Verification items for the finished model (mm, model axes). Face numbers are marked on the shaded views. A direction names the side the tool comes from. Coordinates: 2 decimals unless noted, no trailing zeros. Loops run counter-clockwise (first coordinate to the right, second up) from the corner with the lowest first, then second, coordinate; pieces in that order, holes last. Notation, with made-up numbers: (88.25, 39) - (107.25, 39) arc R32 cw to (107.25, 66) - close; hole circle Ø8 at (-16.75, -11.5). An arc over 180 degrees is marked (long way). One line per item, written item: value. Start each with the question number.
(1) Section check A-A (y = 0). Record the boundary of the cut face in (x, z).
(2) Section check C-C (z = 4.5). Record the boundary of the cut face in (x, y).
(3) Thickness scan on probe 1 along Z at (x, y) = (6, 15.5); probe 2 along Y at (x, z) = (-12, 1); probe 3 along Z at (x, y) = (5.5, 4). Record the ranges inside material, lowest first. Write a range as [from, to].
(4) Set-up check for the marked faces 1 and 2: record each of +Z, -Z, +X, -X, +Y, -Y from which the full face is reachable in a straight line by a thin tool's end or side.
(5) Section check D-D (y = 4). Record the boundary of the cut face in (x, z).
(6) Gauge pin test, flat ends, axial feed: P1, Ø5, axis at x = -8, y = 10, coming from the +Z side; P2, Ø3, axis at x = -11.5, z = -0.5, coming from the -Y side; P3, Ø10, axis at x = -14, y = -12, coming from the -Z side. Record the tip position at first contact, or that the pin passes through.
```python
from build123d import *


with BuildPart() as part:
    # Sketch1 → Revolve1 (revolve)
    with BuildSketch(Plane(origin=(0, 0, 0), x_dir=(0, 0, -1), z_dir=(1, 0, 0)), mode=Mode.PRIVATE) as revolve1_sk:
        with BuildLine():
            Line((8, 0), (8, 6))
            Line((8, 6), (0, 6))
            Line((0, 6), (0, 17.5))
            Line((0, 17.5), (-3.5, 17.5))
            Line((-3.5, 17.5), (-3.5, 18.5))
            Line((-3.5, 18.5), (-6.5, 18.5))
            ThreePointArc((-6.5, 18.5), (-9.117307443, 9.414085192), (-10, 0))
            Line((-10, 0), (8, 0))
        make_face()
    revolve(revolve1_sk.sketch.rotate(Axis((0, 0, -8), (0, 0, -1)), 90), axis=Axis((0, 0, -8), (0, 0, -1)))


solid = part.part
```
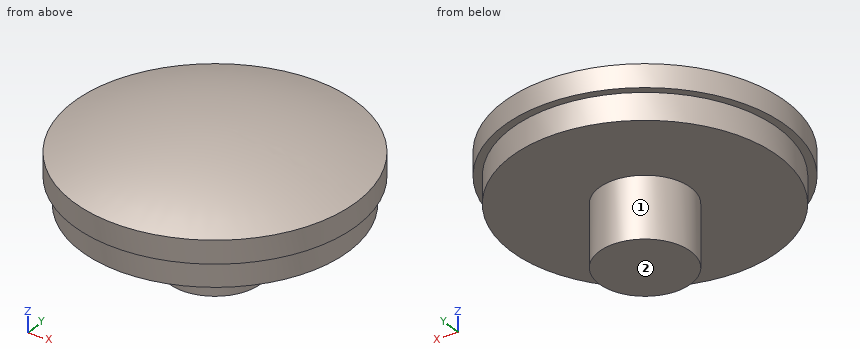
Responses:
1. outline: (-18.5, 3.5) - (-17.5, 3.5) - (-17.5, 0) - (-6, 0) - (-6, -8) - (6, -8) - (6, 0) - (17.5, 0) - (17.5, 3.5) - (18.5, 3.5) - (18.5, 6.5) arc R50.64 ccw to (-18.5, 6.5) - close
2. outline: circle Ø37 at (0, 0)
3. probe 1: z = [0, 7.19]
3. probe 2: y = [-12.74, 12.74]
3. probe 3: z = [0, 9.54]
4. face 1: -Z
4. face 2: -Z, +X, -X, +Y, -Y
5. outline: (-18.06, 3.5) - (-17.04, 3.5) - (-17.04, 0) - (-4.47, 0) - (-4.47, -8) - (4.47, -8) - (4.47, 0) - (17.04, 0) - (17.04, 3.5) - (18.06, 3.5) - (18.06, 6.5) arc R50.48 ccw to (-18.06, 6.5) - close
6. P1: stops at z = 8.94
6. P2: stops at y = -14.3
6. P3: stops at z = 0
